from build123d import *

# Parameters (mm, degrees)
SKETCH1_R           = 1.5
BOSS_EXTRUDE2_DEPTH = 4
SKETCH2_W           = 7.520049523
SKETCH2_H           = 10
BOSS_EXTRUDE3_DEPTH = 3
SKETCH4_W           = 12
SKETCH4_H           = 14
BOSS_EXTRUDE4_DEPTH = 64
CUT_EXTRUDE1_DEPTH  = 61
SKETCH6_W           = 5
SKETCH6_H           = 40
BOSS_EXTRUDE5_DEPTH = 2


with BuildPart() as part:
    # Sketch1 → Boss-Extrude2 (new body)
    with BuildSketch(Plane(origin=(0, 0, 0), x_dir=(1, 0, 0), z_dir=(0, 1, 0))):
        with BuildLine():
            Line((-54.068965517, 20), (-54.068965517, 40))
            Line((-54.068965517, 40), (25.931034483, 40))
            Line((25.931034483, 40), (25.931034483, -20))
            Line((25.931034483, -20), (-54.068965517, -20))
            Line((-54.068965517, -20), (-54.068965517, 0))
            Line((-54.068965517, 0), (-71.068965517, 0))
            ThreePointArc((-71.068965517, 0), (-73.190285861, 0.878679656), (-74.068965517, 3))
            Line((-74.068965517, 3), (-74.068965517, 17))
            ThreePointArc((-74.068965517, 17), (-73.190285861, 19.121320344), (-71.068965517, 20))
            Line((-71.068965517, 20), (-54.068965517, 20))
        make_face()
        with Locations((-50.068965517, 35)):
            Circle(SKETCH1_R, mode=Mode.SUBTRACT)
        with Locations((-44.068965517, 35)):
            Circle(SKETCH1_R, mode=Mode.SUBTRACT)
        with Locations((-50.068965517, -15)):
            Circle(SKETCH1_R, mode=Mode.SUBTRACT)
        with Locations((-44.068965517, -15)):
            Circle(SKETCH1_R, mode=Mode.SUBTRACT)
        with Locations((21.931034483, -15)):
            Circle(SKETCH1_R, mode=Mode.SUBTRACT)
        with Locations((15.931034483, -15)):
            Circle(SKETCH1_R, mode=Mode.SUBTRACT)
        with Locations((15.931034483, 35)):
            Circle(SKETCH1_R, mode=Mode.SUBTRACT)
        with Locations((21.931034483, 35)):
            Circle(SKETCH1_R, mode=Mode.SUBTRACT)
    extrude(amount=BOSS_EXTRUDE2_DEPTH)

    # Sketch2 → Boss-Extrude3 (add)
    with BuildSketch(Plane(origin=(0, 4, 0), x_dir=(1, 0, 0), z_dir=(0, 1, 0))):
        with Locations((-62.530885471, 10)):
            Rectangle(SKETCH2_W, SKETCH2_H)
    extrude(amount=BOSS_EXTRUDE3_DEPTH)

    # Sketch4 → Boss-Extrude4 (add)
    with BuildSketch(Plane(origin=(0, 0, 0), x_dir=(0, 0, -1), z_dir=(1, 0, 0))):
        Polygon((7.602984215, 7), (7.602984215, 17), (0.102984215, 17), (0.102984215, 37), (20.102984215, 37), (20.102984215, 17), (12.602984215, 17), (12.602984215, 7), align=None)
        with Locations((10.102984215, 27)):
            Rectangle(SKETCH4_W, SKETCH4_H, mode=Mode.SUBTRACT)
    extrude(amount=-BOSS_EXTRUDE4_DEPTH)

    # Sketch5 → Cut-Extrude1 (cut)
    with BuildSketch(Plane(origin=(0, 0, 0), x_dir=(0, 0, -1), z_dir=(1, 0, 0))):
        Polygon((0.102984215, 37), (0.102984215, 17), (7.602984215, 17), (7.602984215, 7), (12.602984215, 7), (12.602984215, 17), (20.102984215, 17), (20.102984215, 37), align=None)
    extrude(amount=-CUT_EXTRUDE1_DEPTH, mode=Mode.SUBTRACT)

    # Sketch6 → Boss-Extrude5 (add)
    with BuildSketch(Plane(origin=(0, 37, 0), x_dir=(1, 0, 0), z_dir=(0, 1, 0))):
        with Locations((-62.5, 10)):
            Rectangle(SKETCH6_W, SKETCH6_H)
    extrude(amount=BOSS_EXTRUDE5_DEPTH)


solid = part.part
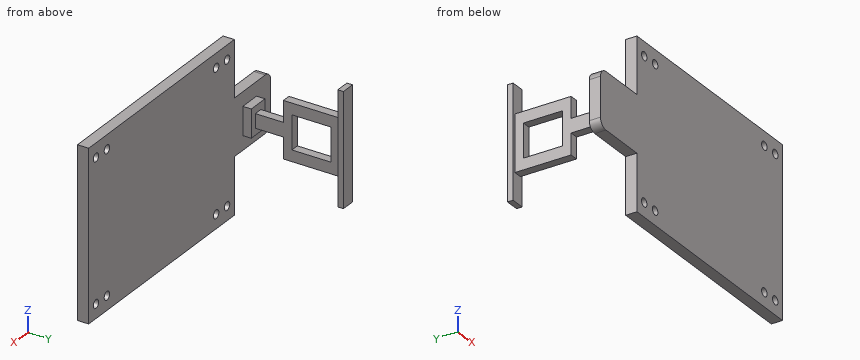
Could you check a few things on this model? Use its own coordinates, in mm. Round coordinates to 2 decimals unless told otherwise and drop trailing zeros. Order: outer loops, then holes, each group sorted by start corner. A loop starts at its lowest first (then second) coordinate and runs counter-clockwise, first axis right, second up. Notation, with made-up numbers: M -38.5,62 L -13.5,62 A24 ccw -13.5,82 Z; hole C 30,24.25 d2. An arc over 180 degrees is marked long. One line per item, written item: value.
(1) Imagine slicing it at B-B (y = 27.5). Write out the boundary of the cut face in (x, z).
Ans:
outline: M -64,-20.1 L -61,-20.1 L -61,-16.1 L -64,-16.1 Z; M -64,-4.1 L -61,-4.1 L -61,-0.1 L -64,-0.1 Z
(2) Imagine slicing it at C-C (z = -6). Write out the boundary of the cut face in (x, y), and give its area (3 significant figures).
Ans:
outline: M -74.07,0 L 25.93,0 L 25.93,4 L -58.77,4 L -58.77,7 L -66.29,7 L -66.29,4 L -74.07,4 Z; M -65,37 L -64,37 L -64,34 L -61,34 L -61,37 L -60,37 L -60,39 L -65,39 Z; M -64,17 L -61,17 L -61,20 L -64,20 Z
area: 451 mm^2
(3) Imagine slicing it at D-D (y = 18). Write out the boundary of the cut face in (x, z).
Ans:
outline: M -64,-20.1 L -61,-20.1 L -61,-0.1 L -64,-0.1 Z
(4) Imagine slicing it at A-A (z = -35). Write out the boundary of the cut face in (x, y).
Ans:
outline: M -54.07,0 L -51.57,0 L -51.57,4 L -54.07,4 Z; M -48.57,0 L -45.57,0 L -45.57,4 L -48.57,4 Z; M -42.57,0 L 14.43,0 L 14.43,4 L -42.57,4 Z; M 17.43,0 L 20.43,0 L 20.43,4 L 17.43,4 Z; M 23.43,0 L 25.93,0 L 25.93,4 L 23.43,4 Z
(5) I need wall thicknesses on line 1 along X through (y, z) = (2.3, 15); line 2 along Y through (x, z) = (4, -28); line 3 along X through (y, z) = (10, -8.5). Which ranges of each line are inside material? Lowest first, please. Write a range as from..to.
Ans:
line 1: x = -54.07..-51.57, -48.57..-45.57, -42.57..14.43, 17.43..20.43, 23.43..25.93
line 2: y = 0..4
line 3: x = -64..-61
(6) I'm going to push flat-ended pins straight in: P1, Ø3.5, axis at y = 6, z = -10.5, coming from the +X side; P2, Ø4.5, axis at x = -59, y = 2.5, coming from the +Z side; P3, Ø12, axis at y = 9, z = -26.5, coming from the -X side; P4, Ø1.5, axis at x = -61.5, z = -8.5, coming from the -Y side. Where does each tip first touch, or does it pass through?
Ans:
P1: stops at x = -58.77
P2: stops at z = 0
P3: stops at x = -54.07
P4: stops at y = 0
